```python
from build123d import *

# Parameters (mm, degrees)
BOSS_EXTRUDE1_DEPTH = 3
SKETCH2_R           = 1.6
CUT_EXTRUDE1_DEPTH  = 10
SKETCH3_R           = 1.5
BOSS_EXTRUDE4_DEPTH = 3


with BuildPart() as part:
    # Sketch1 → Boss-Extrude1 (new body)
    with BuildSketch(Plane.XY):
        with BuildLine():
            Line((38.458853732, -59.570964101), (-38.458853732, -59.570964101))
            ThreePointArc((-38.458853732, -59.570964101), (-48.701494419, -63.813604788), (-44.458853732, -53.570964101))
            Line((-44.458853732, -53.570964101), (-44.458853732, 53.570964101))
            ThreePointArc((-44.458853732, 53.570964101), (-48.701494419, 63.813604788), (-38.458853732, 59.570964101))
            Line((-38.458853732, 59.570964101), (38.458853732, 59.570964101))
            ThreePointArc((38.458853732, 59.570964101), (48.701494419, 63.813604788), (44.458853732, 53.570964101))
            Line((44.458853732, 53.570964101), (44.458853732, -53.570964101))
            ThreePointArc((44.458853732, -53.570964101), (48.701494419, -63.813604788), (38.458853732, -59.570964101))
        make_face()
    extrude(amount=BOSS_EXTRUDE1_DEPTH)

    # Sketch2 → Cut-Extrude1 (cut)
    with BuildSketch(Plane.XY.offset(3)):
        with Locations((-44.458853732, 59.570964101)):
            Circle(SKETCH2_R)
        with Locations((44.458853732, 59.570964101)):
            Circle(SKETCH2_R)
        with Locations((44.458853732, -59.570964101)):
            Circle(SKETCH2_R)
        with Locations((-44.458853732, -59.570964101)):
            Circle(SKETCH2_R)
    extrude(amount=-CUT_EXTRUDE1_DEPTH, mode=Mode.SUBTRACT)

    # Sketch3 → Boss-Extrude4 (add)
    with BuildSketch(Plane.XY.offset(3)):
        with BuildLine():
            Line((19.344784152, 59.570964101), (28.458853732, 59.570964101))
            Line((28.458853732, 59.570964101), (28.458853732, 69.570964101))
            ThreePointArc((28.458853732, 69.570964101), (23.901818942, 74.127998891), (19.344784152, 69.570964101))
            Line((19.344784152, 69.570964101), (19.344784152, 59.570964101))
        make_face()
        with Locations((23.901818942, 69.570964101)):
            Circle(SKETCH3_R, mode=Mode.SUBTRACT)
        with BuildLine():
            Line((-19.344784152, 59.570964101), (-28.458853732, 59.570964101))
            Line((-28.458853732, 59.570964101), (-28.458853732, 69.570964101))
            ThreePointArc((-28.458853732, 69.570964101), (-23.901818942, 74.127998891), (-19.344784152, 69.570964101))
            Line((-19.344784152, 69.570964101), (-19.344784152, 59.570964101))
        make_face()
        with Locations((-23.901818942, 69.570964101)):
            Circle(SKETCH3_R, mode=Mode.SUBTRACT)
    extrude(amount=-BOSS_EXTRUDE4_DEPTH)


solid = part.part
```
Input: part model. Units: mm. Frame: model coordinates. A direction names the side the tool comes from. Give positions to 0.01 mm unless a question says otherwise; leave off trailing zeros. Order: outer loops, then holes, each group sorted by start corner. A loop starts at its lowest first (then second) coordinate and runs counter-clockwise, first axis right, second up. Notation, with made-up numbers: M -21,27.5 L 14,27.5 A20 ccw 14,35.5 Z; hole C -20,-8.5 d5. An arc over 180 degrees is marked long. Return JSON: item names as keys, results as strings.
1) Access query for faces 4 (the face through (44.459, 1, 1)), 5 (the face through (-28.459, 65, 2)), 6 (the face through (1, 5, 0)), 7 (the face through (-44.459, -1, 1)). Directions: +Z, -Z, +X, -X, +Y, -Y. A direction counts if a zero-diameter tool reaches every point of the face in a straight line with its end or side. Return the directions, or none.
Taken from the geometry:
{"face 4": "+Z, -Z, +X", "face 5": "+Z, -Z, +Y", "face 6": "-Z, +X, -X, +Y, -Y", "face 7": "+Z, -Z, -X"}
2) Section query A-A on z = 1.3. Output: boundary loops of the cut face in (x, y), and give its area (3 significant figures).
Taken from the geometry:
{"outline": "M -44.46,-53.57 A6 ccw long -38.46,-59.57 L 38.46,-59.57 A6 ccw long 44.46,-53.57 L 44.46,53.57 A6 ccw long 38.46,59.57 L 28.46,59.57 L 28.46,69.57 A4.56 ccw 19.34,69.57 L 19.34,59.57 L -19.34,59.57 L -19.34,69.57 A4.56 ccw -28.46,69.57 L -28.46,59.57 L -38.46,59.57 A6 ccw long -44.46,53.57 Z; hole C -44.46,-59.57 d3.2; hole C -44.46,59.57 d3.2; hole C -23.9,69.57 d3; hole C 23.9,69.57 d3; hole C 44.46,-59.57 d3.2; hole C 44.46,59.57 d3.2", "area": "11,100 mm2"}
3) Mould query, pull axis Y, two halves, no side actions, for faces 1 (the face through (1, -59.571, 1)), 2 (the face through (19.345, 65, 2)), 3 (the face through (-23.1, 70.84, 1.52)). Classes: released by +Y, released by -Y, zero draft, split by the parting line, or undercut.
Taken from the geometry:
{"face 1": "released by -Y", "face 2": "zero draft", "face 3": "undercut"}
4) Contact query for flat-ended pins moving along their axis: pin 1 (4 mm diameter, centred on x = -23.9, y = 69.57, fed in from -Z); pin 2 (0.9 mm diameter, centred on x = -34, z = 1.5, fed in from +Y); pin 3 (1.5 mm diameter, centred on y = 64, z = 1, fed in from -X); pin 4 (1.5 mm diameter, centred on y = 10, z = 1.5, fed in from +X). Output: stop coordinate, or through.
Taken from the geometry:
{"pin 1": "stops at z = 0", "pin 2": "stops at y = 59.57", "pin 3": "stops at x = -49.2", "pin 4": "stops at x = 44.46"}
5) Section query B-B on y = -12.5. Output: boundary loops of the cut face in (x, z).
Taken from the geometry:
{"outline": "M -44.46,0 L 44.46,0 L 44.46,3 L -44.46,3 Z"}
6) Line query: L1, parallel to X at y = 60.5, z = 2.3; L2, parallel to X at y = -59, z = 2.05; L3, parallel to X at y = -27, z = 1.1. Output: solid intervals per line, ascending. Write a range as [from, to].
Taken from the geometry:
{"L1": "x = [-50.39, -45.76], [-43.16, -38.53], [-28.46, -19.34], [19.34, 28.46], [38.53, 43.16], [45.76, 50.39]", "L2": "x = [-50.43, -45.95], [-42.96, 42.96], [45.95, 50.43]", "L3": "x = [-44.46, 44.46]"}
7) Section query C-C on x = 5.5. Output: boundary loops of the cut face in (y, z).
Taken from the geometry:
{"outline": "M -59.57,0 L 59.57,0 L 59.57,3 L -59.57,3 Z"}
